from build123d import *

# Parameters (mm, degrees)
F0_W     = 23.217392
F0_H     = 21.835592
F1_DEPTH = 10
F2_W     = 26.445957
F2_H     = 27.469668
F3_DEPTH = 25
F4_R     = 5
F5_R     = 5
F6_R     = 2
F6_R_2   = 2.033505
F6_R_3   = 2.079501
F6_R_4   = 1.815846
F7_DEPTH = 25


with BuildPart() as f1:
    # F0 (on Top) → F1 (new body)
    with BuildSketch(Plane.XY):
        Polygon((-6.648776, 53.989464), (-51.648776, 53.989464), (-40.906838, 42.266803), (-17.689446, 42.266803), (-17.689446, 20.431211), (-6.648776, 8.989464), align=None)
        Polygon((-40.906838, 42.266803), (-51.648776, 53.989464), (-51.648776, 8.989464), (-6.648776, 8.989464), (-17.689446, 20.431211), (-40.906838, 20.431211), align=None)
        with Locations((-29.298142, 31.349007)):
            Rectangle(F0_W, F0_H)
    extrude(amount=F1_DEPTH)

    # F2 (on Top) → F3 (cut)
    with BuildSketch(Plane.XY):
        with Locations((-28.950831, 31.422166)):
            Rectangle(F2_W, F2_H)
    extrude(amount=F3_DEPTH, mode=Mode.SUBTRACT)

    # F4
    f4_edges = [f1.edges().sort_by_distance(p)[0] for p in [
        (-51.648776, 8.989464, 5),
        (-51.648776, 53.989464, 5),
        (-6.648776, 53.989464, 5),
        (-6.648776, 8.989464, 5),
    ]]
    fillet(f4_edges, radius=F4_R)

    # F5
    f5_edges = [f1.edges().sort_by_distance(p)[0] for p in [
        (-42.17381, 17.687332, 5),
        (-42.17381, 45.157, 5),
        (-15.727853, 45.157, 5),
        (-15.727853, 17.687332, 5),
    ]]
    fillet(f5_edges, radius=F5_R)

    # F6 (on Top) → F7 (cut)
    with BuildSketch(Plane.XY):
        with Locations((-29.471436, 49.004467)):
            Circle(F6_R)
        with Locations((-46.240133, 31.578172)):
            Circle(F6_R_2)
        with Locations((-29.471436, 14.316277)):
            Circle(F6_R_3)
        with Locations((-11.716344, 31.578172)):
            Circle(F6_R_4)
    extrude(amount=F7_DEPTH, mode=Mode.SUBTRACT)


solid = f1.part
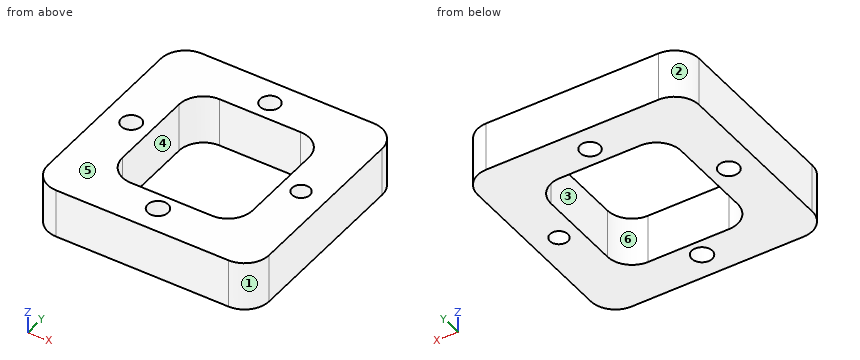
Can you work these out from the model? Positions are in its coordinate system, mm. Face numbers are marked on the shaded views. A direction names the side the tool comes from. Round coordinates to 2 decimals unless told otherwise and drop trailing zeros. Loops run counter-clockwise (first coordinate to the right, second up) from the corner with the lowest first, then second, coordinate; pieces in that order, holes last. Notation, with made-up numbers: (12.25, 32.5) - (56.25, 32.5) arc R30 ccw to (56.25, 63.5) - close; hole circle Ø8 at (-37.5, 78). An arc over 180 degrees is marked (long way). Answer in a Markdown table with one row per item. Add a question column.
Q1. I need wall thicknesses on L1, parallel to Y at x = -34.5, z = 8.75; L2, parallel to X at y = 35.5, z = 0.5; L3, parallel to Y at x = -29, z = 8.25. Which ranges of each line are inside material? Lowest first, please.
Q2. For pin 1 Ø1.5 at (x, y) = (-47, 26) entering from -Z, with a flat end and sliding along its axis, tell me the tip position at first contact or that it passes through.
Q3. Which directions (+Z, -Z, +X, -X, +Y, -Y) give clear straight access to the entire face, cutting with the end or side of a thin tool? Please do the marked faces 5 and 6.
Q4. I want a section at C-C on z = 7.25. List the corners of the cut face in (x, y) for me, and give its area (3 significant figures).
Q5. I want a section at B-B on y = 27.5. List the corners of the cut face in (x, z) for me, and give its area (3 significant figures).
Q6. I want a section at A-A on x = -36. List the corners of the cut face in (y, z) for me.
Q7. We'd pull the mould along X, two halves only. Please class the marked faces 1, 2, 3 and 4: pulls with the +X half, pulls with the -X half, needs draft (parallel to the pull), parting line crosses it, or undercut.
A:
| question | item | result |
|---|---|---|
| 1 | L1 | 8.99 to 17.69, 45.16 to 53.99 |
| 1 | L2 | -51.65 to -42.17, -15.73 to -6.65 |
| 1 | L3 | 8.99 to 12.29, 16.34 to 17.69, 45.16 to 47.06, 50.95 to 53.99 |
| 2 | pin 1 | z = 0 |
| 3 | face 5 | +Z, +X, -X, +Y, -Y |
| 3 | face 6 | +Z, -Z |
| 4 | outline | (-51.65, 13.99) arc R5 ccw to (-46.65, 8.99) - (-11.65, 8.99) arc R5 ccw to (-6.65, 13.99) - (-6.65, 48.99) arc R5 ccw to (-11.65, 53.99) - (-46.65, 53.99) arc R5 ccw to (-51.65, 48.99) - close; hole circle Ø4.07 at (-46.24, 31.58); hole (-42.17, 22.69) arc R5 ccw to (-37.17, 17.69) - (-20.73, 17.69) arc R5 ccw to (-15.73, 22.69) - (-15.73, 40.16) arc R5 ccw to (-20.73, 45.16) - (-37.17, 45.16) arc R5 ccw to (-42.17, 40.16) - close; hole circle Ø4.16 at (-29.47, 14.32); hole circle Ø4 at (-29.47, 49); hole circle Ø3.63 at (-11.72, 31.58) |
| 4 | area | 1,250 mm^2 |
| 5 | outline | (-51.65, 0) - (-42.17, 0) - (-42.17, 10) - (-51.65, 10) - close; (-15.73, 0) - (-6.65, 0) - (-6.65, 10) - (-15.73, 10) - close |
| 5 | area | 186 mm^2 |
| 6 | outline | (8.99, 0) - (17.69, 0) - (17.69, 10) - (8.99, 10) - close; (45.16, 0) - (53.99, 0) - (53.99, 10) - (45.16, 10) - close |
| 7 | face 1 | pulls with the +X half |
| 7 | face 2 | pulls with the -X half |
| 7 | face 3 | undercut |
| 7 | face 4 | undercut |
